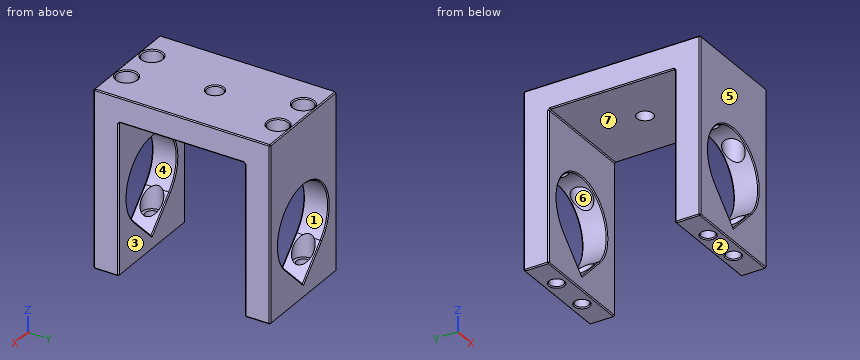
```python
from build123d import *

# Parameters (mm, degrees)
SKETCH001_W     = 42
SKETCH001_H     = 70
PAD001_DEPTH    = 70
POCKET_DEPTH    = 70
SKETCH003_W     = 42
SKETCH003_H     = 50
POCKET001_DEPTH = 60
SKETCH004_R     = 3.2
POCKET002_DEPTH = 10
SKETCH005_R     = 2.7
POCKET003_DEPTH = 70
SKETCH007_R     = 4
POCKET004_DEPTH = 62
CHAMFER001_SIZE = 0.4


with BuildPart() as part:
    # Sketch001 → Pad001 (new body)
    with BuildSketch(Plane.XY):
        Rectangle(SKETCH001_W, SKETCH001_H)
    extrude(amount=PAD001_DEPTH)

    # Sketch002 (on Face3 of Pad001) → Pocket (cut)
    with BuildSketch(Plane.XZ.offset(35)):
        with BuildLine():
            ThreePointArc((11.313708, 16.686292), (0, 44), (-11.313708, 16.686292))
            Line((-11.313708, 16.686292), (0, 5.372583))
            Line((0, 5.372583), (11.313708, 16.686292))
        make_face()
    extrude(amount=-POCKET_DEPTH, mode=Mode.SUBTRACT)

    # Sketch003 (on Face3 of Pocket) → Pocket001 (cut)
    with BuildSketch(Plane(origin=(0, 0, 0), x_dir=(1, 0, 0), z_dir=(0, 0, -1))):
        Rectangle(SKETCH003_W, SKETCH003_H)
    extrude(amount=-POCKET001_DEPTH, mode=Mode.SUBTRACT)

    # Sketch004 (on Face4 of Pocket001) → Pocket002 (cut)
    with BuildSketch(Plane.XY.offset(70)):
        Circle(SKETCH004_R)
    extrude(amount=-POCKET002_DEPTH, mode=Mode.SUBTRACT)

    # Sketch005 (on Face9 of Pocket001) → Pocket003 (cut)
    with BuildSketch(Plane(origin=(0, 0, 0), x_dir=(1, 0, 0), z_dir=(0, 0, -1))):
        with Locations((-8, 30)):
            Circle(SKETCH005_R)
        with Locations((8, 30)):
            Circle(SKETCH005_R)
        with Locations((-8, -30)):
            Circle(SKETCH005_R)
        with Locations((8, -30)):
            Circle(SKETCH005_R)
    extrude(amount=-POCKET003_DEPTH, mode=Mode.SUBTRACT)

    # Sketch007 (on Face4 of Pocket003) → Pocket004 (cut)
    with BuildSketch(Plane.XY.offset(70)):
        with Locations((-8, 30)):
            Circle(SKETCH007_R)
        with Locations((8, 30)):
            Circle(SKETCH007_R)
        with Locations((8, -30)):
            Circle(SKETCH007_R)
        with Locations((-8, -30)):
            Circle(SKETCH007_R)
    extrude(amount=-POCKET004_DEPTH, mode=Mode.SUBTRACT)

    # Chamfer001
    chamfer001_edges = [part.edges().sort_by_distance(p)[0] for p in [
        (0, 35, 70),
        (-21, 0, 70),
        (21, 0, 70),
        (0, -35, 70),
        (-12, -30, 70),
        (4, -30, 70),
        (-12, 30, 70),
        (-3.2, 0, 70),
        (4, 30, 70),
        (21, -35, 35),
        (0, -35, 0),
        (-21, -35, 35),
        (0, -35, 44),
        (-5.656854, -35, 11.029437),
        (5.656854, -35, 11.029437),
        (-21, -30, 0),
        (-21, -25, 30),
        (-21, 0, 60),
        (-21, 25, 30),
        (-21, 30, 0),
        (-21, 35, 35),
        (0, 35, 0),
        (21, 35, 35),
        (5.656854, 35, 11.029437),
        (-5.656854, 35, 11.029437),
        (0, 35, 44),
        (21, 30, 0),
        (21, 25, 30),
        (21, 0, 60),
        (21, -25, 30),
        (21, -30, 0),
        (0, -25, 0),
        (0, -25, 60),
        (-5.656854, -25, 11.029437),
        (0, -25, 44),
        (5.656854, -25, 11.029437),
        (0, 25, 0),
        (0, 25, 60),
        (0, 25, 44),
        (-5.656854, 25, 11.029437),
        (5.656854, 25, 11.029437),
        (5.3, -30, 0),
        (-10.7, -30, 0),
        (-10.7, 30, 0),
        (5.3, 30, 0),
    ]]
    chamfer(chamfer001_edges, length=CHAMFER001_SIZE)


solid = part.part
```
CAD build for the part. Positions are in the model's coordinates, mm. Face numbers are marked on the shaded views. A direction names the side the tool comes from. Coordinates: 2 decimals unless noted, no trailing zeros. Order: outer loops, then holes, each group sorted by start corner. A loop starts at its lowest first (then second) coordinate and runs counter-clockwise, first axis right, second up.
(1) Mould opens along Z. For the marked faces 1, 2, 3 and 4 say: released by +Z, released by -Z, zero draft, split by the parting line, or undercut.
Solution:
face 1: undercut
face 2: released by -Z
face 3: zero draft
face 4: undercut
(2) Saw through at B-B, the plane y = 16. Write the cut outline in (x, z).
Solution:
outline: (-21, 60.4) - (-20.6, 60) - (20.6, 60) - (21, 60.4) - (21, 69.6) - (20.6, 70) - (-20.6, 70) - (-21, 69.6) - close
(3) Saw through at C-C, the plane x = -6.5. Count the separate pieces of the cut face and the enclosed holes in it, and give its area (3 significant figures).
Solution:
separate pieces: 7
enclosed holes: 0
area: 748 mm2
(4) Pin check, flat tips, straight feed: pin 1 Ø10.5 at (x, y) = (-8, 30) entering from +Z; pin 2 Ø4 at (x, y) = (-8.5, -31) entering from +Z; pin 3 Ø5 at (x, y) = (8, -30) entering from +Z; pin 4 Ø3 at (x, y) = (8.5, -16) entering from -Z. Stop position of each tip, or through.
Solution:
pin 1: stops at z = 70
pin 2: stops at z = 8
pin 3: passes through
pin 4: stops at z = 60
(5) Drill centre lines: L1, parallel to Y at x = 8, z = 11; L2, parallel to X at y = -30, z = 62.5; L3, parallel to Y at x = 15, z = 21. Where is each one in solid material? Low to high.
Solution:
L1: y = -35 to -34, -26 to -25, 25 to 26, 34 to 35
L2: x = -21 to -12, -4 to 4, 12 to 21
L3: y = -35 to -25, 25 to 35
(6) Which spindle directions (+Z, -Z, +X, -X, +Y, -Y) get a long thin tool onto all of the face, cutting with end or side? Do the marked faces 5, 6 and 7. Say none if no direction does.
Solution:
face 5: +Z, -Z, +X, -X, -Y
face 6: +Z
face 7: -Z, +X, -X
(7) Saw through at A-A, the plane z = 47.5. Write the cut outline in (x, y), and give its area (3 significant figures).
Solution:
outline: (-21, -34.6) - (-20.6, -35) - (20.6, -35) - (21, -34.6) - (21, -25.4) - (20.6, -25) - (-20.6, -25) - (-21, -25.4) - close; (-21, 25.4) - (-20.6, 25) - (20.6, 25) - (21, 25.4) - (21, 34.6) - (20.6, 35) - (-20.6, 35) - (-21, 34.6) - close; hole circle Ø8 at (-8, -30); hole circle Ø8 at (-8, 30); hole circle Ø8 at (8, -30); hole circle Ø8 at (8, 30)
area: 638 mm2
